Design review of the part built by this model. Coordinates are the model's own, in mm. A direction names the side the tool comes from. Coordinates: 2 decimals unless noted, no trailing zeros. Write each loop counter-clockwise with the first axis right and the second up, starting at its lowest first coordinate (ties: lowest second). Pieces come first, ordered by that corner, then holes.
Q1. The part is to be moulded in two halves that separate along X. For faces 1 (the flat face through (-28.5, 0, 0)), 2 (the cylindrical face through (-23.6, 10.9, 0.4)), 3 (the flat face through (124.5, 0, 0)), 4 (the flat face through (0, -19, 0)), say which applies: released by +X, released by -X, zero draft, split by the parting line, or undercut.
Q2. For L1, parallel to Y at x = 23.5, z = -2; L2, parallel to X at y = -11, z = 1.75; L3, parallel to X at y = -0.5, z = 4.25, list the stretches that pass through material, from the lowest coordinate up.
Q3. Take a section at B-B, the plane z = -3.5. Write out the cut boundary in (x, y), plus the area to 3 significant figures.
Q4. Take a section at A-A, the plane y = -12.5. State how many separate pieces and enclosed holes the cut face has, plus the area to 3 significant figures.
Q5. For pin 1 Ø2 at (x, z) = (57.5, -3) entering from +Y; pin 2 Ø3.5 at (x, y) = (-23.5, -23.5) entering from -Z; pin 3 Ø5 at (x, z) = (106, 3.5) entering from -Y; pin 4 Ø5 at (x, y) = (23.5, 23.5) entering from -Z, all flat-tipped, find the tip position at first contact; note any pin that passes through.
Q6. Take a section at D-D, the plane x = 57. Write out the cut boundary in (y, z).
Q7. Take a section at C-C, the plane y = 0. Write out the cut boundary in (x, z), plus the area to 3 significant figures.
Q8. For faces 5 (the flat face through (-19, 0, 0)), 6 (the cylindrical face through (-20.55, 26.2, -2.73)), 7 (the flat face through (76, -22.5, 0)), list the 3-axis set-ups (+Z, -Z, +X, -X, +Y, -Y) from which the entire face can be reached by the end or side of a thin tool; tool diameter is ignored.
from build123d import *

# Parameters (mm, degrees)
EXTRUDE_1_DEPTH              = 5
SKETCH_6_R                   = 10
CUT_EXTRUDE_1530_DEPTH       = 10
SKETCH_19_R                  = 12
CUT_EXTRUDE_1946_DEPTH       = 5
HOLE_WIZARD_8_5_8_5_1_D      = 8.5
HOLE_WIZARD_1_D              = 4.5
HOLE_WIZARD_1_CBORE_D        = 8
HOLE_WIZARD_1_CBORE_DEPTH    = 4.6
FILLET_1_R                   = 5
CHAMFER_1_SIZE               = 5
CHAMFER_2_SIZE               = 0.2
HOLE_WIZARD_M4_1_D           = 3.3
HOLE_WIZARD_M4_1_DEPTH       = 15.5
HOLE_WIZARD_M4_1_CSINK_D     = 4.05
HOLE_WIZARD_M4_1_CSINK_ANGLE = 120
SKETCH_22_W                  = 38
SKETCH_22_H                  = 38
CUT_EXTRUDE_1_DEPTH          = 10
FILLET_2_R                   = 5


with BuildPart() as part:
    # 草图1 → 凸台-拉伸1 (new body, symmetric)
    with BuildSketch(Plane.XY):
        Polygon((28.5, 28.5), (-28.5, 28.5), (-28.5, -28.5), (28.5, -28.5), (34.5, -22.5), (124.5, -22.5), (124.5, 22.5), (34.5, 22.5), align=None)
    extrude(amount=EXTRUDE_1_DEPTH, both=True)

    # 草图6 → Cut-Extrude 1530 (cut)
    with BuildSketch(Plane.XY.offset(5)):
        Circle(SKETCH_6_R)
    extrude(amount=-CUT_EXTRUDE_1530_DEPTH, mode=Mode.SUBTRACT)

    # 草图19 → Cut-Extrude 1946 (cut)
    with BuildSketch(Plane(origin=(0, 0, -5), x_dir=(-1, 0, 0), z_dir=(0, 0, -1))):
        Circle(SKETCH_19_R)
    extrude(amount=-CUT_EXTRUDE_1946_DEPTH, mode=Mode.SUBTRACT)

    # Ø8.5 (8.5) 直径孔1 (through all)
    with Locations(Plane.XY.offset(5)):
        with Locations((57, 0), (102, 0)):
            Hole(HOLE_WIZARD_8_5_8_5_1_D / 2)

    # 打孔尺寸(%根据)内六角圆柱头螺钉的类型1 (through all)
    with Locations(Plane(origin=(0, 0, -5), x_dir=(-1, 0, 0), z_dir=(0, 0, -1))):
        with Locations((-23.5, 23.5), (23.5, 23.5), (23.5, -23.5), (-23.5, -23.5)):
            CounterBoreHole(HOLE_WIZARD_1_D / 2, HOLE_WIZARD_1_CBORE_D / 2, HOLE_WIZARD_1_CBORE_DEPTH)

    # 圆角1
    fillet_1_edges = [part.edges().sort_by_distance(p)[0] for p in [
        (-28.5, -28.5, 0),
        (-28.5, 28.5, 0),
    ]]
    fillet(fillet_1_edges, radius=FILLET_1_R)

    # 倒角1
    chamfer_1_edges = [part.edges().sort_by_distance(p)[0] for p in [
        (124.5, 22.5, 0),
        (124.5, -22.5, 0),
    ]]
    chamfer(chamfer_1_edges, length=CHAMFER_1_SIZE)

    # 倒角2
    chamfer_2_edges = [part.edges().sort_by_distance(p)[0] for p in [
        (12, 0, -5),
    ]]
    chamfer(chamfer_2_edges, length=CHAMFER_2_SIZE)

    # M4 螺纹孔1
    with Locations(Plane.ZY.offset(28.5)):
        with Locations((0, 12.5), (0, -12.5)):
            CounterSinkHole(HOLE_WIZARD_M4_1_D / 2, HOLE_WIZARD_M4_1_CSINK_D / 2, depth=HOLE_WIZARD_M4_1_DEPTH, counter_sink_angle=HOLE_WIZARD_M4_1_CSINK_ANGLE)

    # 草图22 → 切除-拉伸1 (cut)
    with BuildSketch(Plane(origin=(0, 0, -5), x_dir=(-1, 0, 0), z_dir=(0, 0, -1))):
        Rectangle(SKETCH_22_W, SKETCH_22_H)
    extrude(amount=-CUT_EXTRUDE_1_DEPTH, mode=Mode.SUBTRACT)

    # 圆角2
    fillet_2_edges = [part.edges().sort_by_distance(p)[0] for p in [
        (-19, 19, 0),
        (-19, -19, 0),
        (19, -19, 0),
        (19, 19, 0),
    ]]
    fillet(fillet_2_edges, radius=FILLET_2_R)


solid = part.part
Responses:
1. face 1: released by -X
1. face 2: zero draft
1. face 3: released by +X
1. face 4: undercut
2. L1: y = -28.5 to -27.5, -19.5 to 19.5, 27.5 to 28.5
2. L2: x = -28.5 to -19, 19 to 124.5
2. L3: x = -28.5 to -19, 19 to 52.78, 61.22 to 97.78, 106.22 to 124.5
3. outline: (-28.5, -23.5) arc R5 ccw to (-23.5, -28.5) - (28.5, -28.5) - (34.5, -22.5) - (119.5, -22.5) - (124.5, -17.5) - (124.5, 17.5) - (119.5, 22.5) - (34.5, 22.5) - (28.5, 28.5) - (-23.5, 28.5) arc R5 ccw to (-28.5, 23.5) - close; hole circle Ø8 at (-23.5, -23.5); hole circle Ø8 at (-23.5, 23.5); hole (-19, -14) arc R5 ccw to (-14, -19) - (14, -19) arc R5 ccw to (19, -14) - (19, 14) arc R5 ccw to (14, 19) - (-14, 19) arc R5 ccw to (-19, 14) - close; hole circle Ø8 at (23.5, -23.5); hole circle Ø8 at (23.5, 23.5); hole circle Ø8.5 at (57, 0); hole circle Ø8.5 at (102, 0)
3. area: 5,830 mm2
4. separate pieces: 3
4. enclosed holes: 0
4. area: 1,120 mm2
5. pin 1: stops at y = 22.5
5. pin 2: passes through
5. pin 3: stops at y = -22.5
5. pin 4: stops at z = -0.4
6. outline: (-22.5, -5) - (-4.25, -5) - (-4.25, 5) - (-22.5, 5) - close; (4.25, -5) - (22.5, -5) - (22.5, 5) - (4.25, 5) - close
7. outline: (-28.5, -5) - (-19, -5) - (-19, 5) - (-28.5, 5) - close; (19, -5) - (52.75, -5) - (52.75, 5) - (19, 5) - close; (61.25, -5) - (97.75, -5) - (97.75, 5) - (61.25, 5) - close; (106.25, -5) - (124.5, -5) - (124.5, 5) - (106.25, 5) - close
7. area: 980 mm2
8. face 5: +Z, -Z
8. face 6: -Z
8. face 7: +Z, -Z, +X, -Y
